from build123d import *

# Parameters (mm, degrees)
F0_R     = 64.725
F1_DEPTH = 15
F2_R     = 52.725
F2_R_2   = 48.225
F3_DEPTH = 11
F4_R     = 41.225
F5_DEPTH = 10
F7_DEPTH = 5
F8_D     = 6.7564


with BuildPart() as f1:
    # F0 (on Top) → F1 (new body)
    with BuildSketch(Plane.XY):
        Circle(F0_R)
    extrude(amount=F1_DEPTH)

    # F2 (on face) → F3 (cut)
    with BuildSketch(Plane.XY.offset(15)):
        Circle(F2_R)
        Circle(F2_R_2, mode=Mode.SUBTRACT)
    extrude(amount=-F3_DEPTH, mode=Mode.SUBTRACT)

    # F4 (on face) → F5 (cut)
    with BuildSketch(Plane(origin=(0, 0, 0), x_dir=(1, 0, 0), z_dir=(0, 0, -1))):
        Circle(F4_R)
    extrude(amount=-F5_DEPTH, mode=Mode.SUBTRACT)

    # F6 (on face) → F7 (cut, through all)
    with BuildSketch(Plane(origin=(0, 0, 10), x_dir=(1, 0, 0), z_dir=(0, 0, -1))):
        with BuildLine():
            ThreePointArc((0, 12.2501222179), (2.2276802059, 12.0458679743), (4.3810732942, 11.4399165707))
            Line((4.3810732942, 11.4399165707), (13.2776884508, 36.3189443658))
            ThreePointArc((13.2776884508, 36.3189443658), (6.7421083146, 38.0776404983), (0, 38.6699202281))
            Line((0, 38.6699202281), (0, 12.2501222179))
        make_face()
        with BuildLine():
            Line((10.7095334794, 5.9473848881), (33.5166668905, 19.28719189))
            ThreePointArc((33.5166668905, 19.28719189), (29.6405901277, 24.8354212231), (24.8565455902, 29.6228775066))
            Line((24.8565455902, 29.6228775066), (7.8742267788, 9.3841380525))
            ThreePointArc((7.8742267788, 9.3841380525), (9.4494367246, 7.7957449895), (10.7095334794, 5.9473848881))
        make_face()
        with BuildLine():
            Line((12.0268839264, -2.3279942814), (38.0728243958, -6.7692520245))
            ThreePointArc((38.0728243958, -6.7692520245), (38.6699104016, -0.0275676574), (38.082437249, 6.7149611781))
            Line((38.082437249, 6.7149611781), (12.0640153355, 2.1272113993))
            ThreePointArc((12.0640153355, 2.1272113993), (12.249696781, -0.1020937159), (12.0268839264, -2.3279942814))
        make_face()
        with BuildLine():
            Line((7.7167217203, -9.5140790539), (24.8142842341, -29.6582876849))
            ThreePointArc((24.8142842341, -29.6582876849), (29.6051498304, -24.8776573246), (33.4891332798, -19.334960114))
            Line((33.4891332798, -19.334960114), (10.6089170402, -6.1250611089))
            ThreePointArc((10.6089170402, -6.1250611089), (9.3181875734, -7.952161637), (7.7167217203, -9.5140790539))
        make_face()
        with BuildLine():
            Line((-0.2041803405, -12.2484204999), (-0.0551353009, -38.6698809223))
            ThreePointArc((-0.0551353009, -38.6698809223), (6.687810629, -38.0872146453), (13.2258916588, -36.3378386847))
            Line((13.2258916588, -36.3378386847), (4.1897885567, -11.5113494519))
            ThreePointArc((4.1897885567, -11.5113494519), (2.0265948401, -12.0813247497), (-0.2041803405, -12.2484204999))
        make_face()
        with BuildLine():
            Line((-8.0295441508, -9.2515898679), (-24.8987564158, -29.5874071083))
            ThreePointArc((-24.8987564158, -29.5874071083), (-19.3588294925, -33.4753409412), (-13.2258916588, -36.3378386847))
            Line((-13.2258916588, -36.3378386847), (-4.1897885567, -11.5113494519))
            ThreePointArc((-4.1897885567, -11.5113494519), (-6.213264142, -10.5575017431), (-8.0295441508, -9.2515898679))
        make_face()
        with BuildLine():
            Line((-12.0977950145, -1.9258375168), (-38.0919726849, -6.660656681))
            ThreePointArc((-38.0919726849, -6.660656681), (-36.347258145, -13.1999831737), (-33.4891332798, -19.334960114))
            Line((-33.4891332798, -19.334960114), (-10.6089170402, -6.1250611089))
            ThreePointArc((-10.6089170402, -6.1250611089), (-11.5458677793, -4.0937063373), (-12.0977950145, -1.9258375168))
        make_face()
        with BuildLine():
            Line((-10.5053531389, 6.3010356118), (-33.4615315896, 19.3826890323))
            ThreePointArc((-33.4615315896, 19.3826890323), (-36.3284007567, 13.2517934222), (-38.082437249, 6.7149611781))
            Line((-38.082437249, 6.7149611781), (-12.0640153355, 2.1272113993))
            ThreePointArc((-12.0640153355, 2.1272113993), (-11.4760315646, 4.2855797602), (-10.5053531389, 6.3010356118))
        make_face()
        with BuildLine():
            Line((-3.9973397756, 11.5795841493), (-13.1740679801, 36.3566591329))
            ThreePointArc((-13.1740679801, 36.3566591329), (-19.3110809092, 33.5029085986), (-24.8565455902, 29.6228775066))
            Line((-24.8565455902, 29.6228775066), (-7.8742267788, 9.3841380525))
            ThreePointArc((-7.8742267788, 9.3841380525), (-6.036432639, 10.6595954589), (-3.9973397756, 11.5795841493))
        make_face()
    extrude(amount=-F7_DEPTH, mode=Mode.SUBTRACT)

    # F8 (through all)
    with Locations(Plane(origin=(0, 0, 10), x_dir=(1, 0, 0), z_dir=(0, 0, -1))):
        with Locations((0, 0)):
            Hole(F8_D / 2)


solid = f1.part
Geometry: final body of the model. Coordinates: model frame, mm. A direction names the side the tool comes from. Give positions to 0.01 mm unless a question says otherwise; leave off trailing zeros. Write each loop counter-clockwise with the first axis right and the second up, starting at its lowest first coordinate (ties: lowest second). Pieces come first, ordered by that corner, then holes. Notation, with made-up numbers: M 33.25,7 L 90.25,7 A32 cw 90.25,40 Z; hole C 19,21.5 d11. An arc over 180 degrees is marked long. Answer in a Markdown table with one row per item. Add a question column.
(1) First-contact query: pin 1 (3 mm diameter, centred on y = -17.5, z = 5, fed in from +X); pin 2 (6 mm diameter, centred on y = 37.5, z = 8, fed in from +X); pin 3 (1.5 mm diameter, centred on x = -45, z = 7.5, fed in from +Y); pin 4 (6 mm diameter, centred on x = 28, y = 29.5, fed in from -Z). Flat tips, straight axial feed; report the tip coordinate or a pass-through.
(2) Ray query, line 1 (Y direction, x = -1, z = 9); line 2 (X direction, y = -28, z = 6.25); line 3 (X direction, y = -22, z = 11). Return the intervals inside material, ascending.
(3) Section B-B on z = 5.5. Return loops of the section in (x, y) (3 decimals), and give its area (3 significant figures).
(4) Section A-A on y = 0. Return loops of the section in (x, z) (3 decimals).
(5) Mould query, pull axis Y, two halves, no side actions, for faces 3 (the cylindrical face through (-36.296, -13.341, 12.465)), 4 (the flat face through (-1, -42, 0)), 5 (the cylindrical face through (-14.031, -63.186, 7.395)). Classes: +Y half, -Y half, draft (parallel to the pull), parting line (faces both ways), or undercut.
(6) Reachability of faces 1 (the flat face through (-24.91, 4.26, 12.46)), 2 (the cylindrical face through (-6.864, 52.276, 9.577)) from +Z, -Z, +X, -X, +Y, -Y: full face, straight path, thin tool, end or side. Return the list, or none.
(7) Section C-C on y = 44. Return loops of the section in (x, z), and give its area (3 significant figures).
Result set:
| question | item | result |
|---|---|---|
| 1 | pin 1 | stops at x = 62.72 |
| 1 | pin 2 | stops at x = 54.76 |
| 1 | pin 3 | stops at y = 47.24 |
| 1 | pin 4 | stops at z = 0 |
| 2 | line 1 | y = -64.72 to -52.72, -48.21 to -41.21, 41.21 to 48.21, 52.72 to 64.72 |
| 2 | line 2 | x = -58.36 to -44.68, -39.26 to -30.26, 30.26 to 39.26, 44.68 to 58.36 |
| 2 | line 3 | x = -60.87 to -47.92, -42.91 to -18.46, -7.86 to 0, 8.16 to 18.46, 31.8 to 42.91, 47.92 to 60.87 |
| 3 | outline | C 0,0 d129.45; C 0,0 d96.45; hole C 0,0 d105.45; hole C 0,0 d82.45 |
| 3 | area | 6,390 mm^2 |
| 4 | outline | M -64.725,0 L -41.225,0 L -41.225,10 L -3.378,10 L -3.378,15 L -48.225,15 L -48.225,4 L -52.725,4 L -52.725,15 L -64.725,15 Z; M 3.378,10 L 12.25,10 L 12.25,15 L 3.378,15 Z; M 38.67,10 L 41.225,10 L 41.225,0 L 64.725,0 L 64.725,15 L 52.725,15 L 52.725,4 L 48.225,4 L 48.225,15 L 38.67,15 Z |
| 5 | face 3 | undercut |
| 5 | face 4 | draft |
| 5 | face 5 | parting line |
| 6 | face 1 | +Z, -Z |
| 6 | face 2 | +Z |
| 7 | outline | M -47.47,0 L 47.47,0 L 47.47,15 L 29.05,15 L 29.05,4 L 19.74,4 L 19.74,15 L -19.74,15 L -19.74,4 L -29.05,4 L -29.05,15 L -47.47,15 Z |
| 7 | area | 1,220 mm^2 |
